Verification items for the finished model (mm, model axes). Face numbers are marked on the shaded views. Give positions to 0.01 mm unless a question says otherwise; leave off trailing zeros. Loops run counter-clockwise (first coordinate to the right, second up) from the corner with the lowest first, then second, coordinate; pieces in that order, holes last. Notation, with made-up numbers: (89, 55) -> (126, 55) arc R23 cw to (126, 64) -> close; hole circle Ø7 at (-19.75, 65). An arc over 180 degrees is marked (long way). Answer in a Markdown table with one row per item. Add a question column.
Q1. Material ranges on probe 1 along X at (y, z) = (16.5, -7.45); probe 2 along Z at (x, y) = (1.5, 26); probe 3 along X at (y, z) = (33, -3.4), recorded low to high.
Q2. Gauge pin test, flat ends, axial feed: P1, Ø3, axis at x = 1, y = 31.5, coming from the -Z side; P2, Ø0.8, axis at x = 0.5, z = -6.5, coming from the -Y side; P3, Ø1.1, axis at x = 6, z = -3.5, coming from the +Y side. Record the tip position at first contact, or that the pin passes through.
Q3. Section check C-C on z = -7.45. Enter the section's corners in (x, y), and give its area (3 significant figures).
Q4. Section check A-A on y = 17. Enter the section's corners in (x, z), and give its area (3 significant figures).
Q5. Section check B-B on x = -9. Enter the section's corners in (y, z).
Q6. Release check for a two-part mould opening along Z. For the marked faces 1 and 2 record: pulls with the +Z half, pulls with the -Z half, needs draft (parallel to the pull), parting line crosses it, or undercut.
```python
from build123d import *

# Parameters (mm, degrees)
SKETCH_W        = 41.5
SKETCH_H        = 36
PAD_DEPTH       = 6
POCKET_DEPTH    = 5
SKETCH002_W     = 19.5
SKETCH002_H     = 8
POCKET001_DEPTH = 6.001
POCKET002_DEPTH = 1
SKETCH005_W     = 1
SKETCH005_H     = 19
PAD001_DEPTH    = 4
PAD002_DEPTH    = 10
SKETCH007_W     = 52.700282
SKETCH007_H     = 20.841337
POCKET003_DEPTH = 41.501
SKETCH008_W     = 1
SKETCH008_H     = 18
PAD003_DEPTH    = 4


with BuildPart() as part:
    # Sketch → Pad (new body)
    with BuildSketch(Plane.XY):
        with Locations((-0.25, 18)):
            Rectangle(SKETCH_W, SKETCH_H)
    extrude(amount=PAD_DEPTH)

    # Sketch001 (on Face6 of Pad) → Pocket (cut)
    with BuildSketch(Plane.XY.offset(6)):
        Polygon((-19, 2), (18.5, 2), (18.5, 26), (-1, 26), (-1, 34), (-19, 34), align=None)
    extrude(amount=-POCKET_DEPTH, mode=Mode.SUBTRACT)

    # Sketch002 (on Face5 of Pocket) → Pocket001 (cut, through all)
    with BuildSketch(Plane.XY.offset(6)):
        with Locations((10.75, 32)):
            Rectangle(SKETCH002_W, SKETCH002_H)
    extrude(amount=-POCKET001_DEPTH, mode=Mode.SUBTRACT)

    # Sketch004 (on Face5 of Pocket001) → Pocket002 (cut)
    with BuildSketch(Plane.XY.offset(6)):
        Polygon((-20, 35), (0, 35), (0, 27), (19.5, 27), (19.5, 1), (-20, 1), align=None)
    extrude(amount=-POCKET002_DEPTH, mode=Mode.SUBTRACT)

    # Sketch005 (on Face22 of Pocket002) → Pad001 (join)
    with BuildSketch(Plane.XY.offset(1)):
        with Locations((-0.5, 16.5)):
            Rectangle(SKETCH005_W, SKETCH005_H)
    extrude(amount=PAD001_DEPTH)

    # Sketch006 (on Face5 of Pad001) → Pad002 (join)
    with BuildSketch(Plane.XY.offset(6)):
        Polygon((-20, 35), (0, 35), (0, 27), (19.5, 27), (19.5, 1), (-20, 1), align=None)
    extrude(amount=-PAD002_DEPTH)

    # Sketch007 (on Face2 of Pad002) → Pocket003 (cut, through all)
    with BuildSketch(Plane(origin=(-21, 0, 0), x_dir=(0, -1, 0), z_dir=(-1, 0, 0))):
        with Locations((-14.885127, 7.420668)):
            Rectangle(SKETCH007_W, SKETCH007_H)
    extrude(amount=-POCKET003_DEPTH, mode=Mode.SUBTRACT)

    # Sketch008 (on Face4 of Pocket003) → Pad003 (join)
    with BuildSketch(Plane(origin=(0, 0, -4), x_dir=(1, 0, 0), z_dir=(0, 0, -1))):
        with Locations((0.5, -16)):
            Rectangle(SKETCH008_W, SKETCH008_H)
    extrude(amount=PAD003_DEPTH)


solid = part.part
```
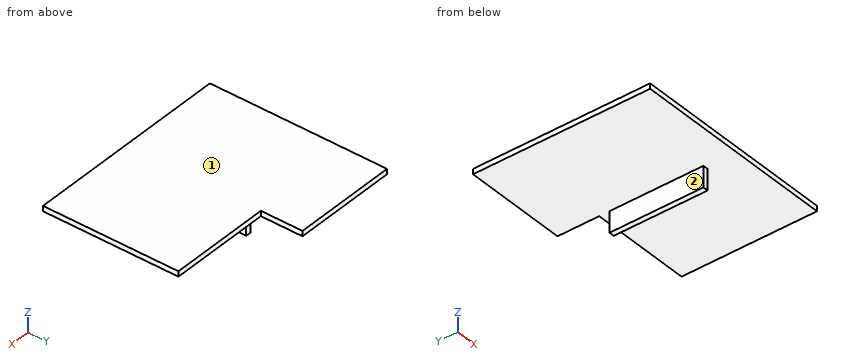
Taken from the geometry:
| question | item | result |
|---|---|---|
| 1 | probe 1 | x = 0 to 1 |
| 1 | probe 2 | z = -4 to -3 |
| 1 | probe 3 | x = -20 to 0 |
| 2 | P1 | stops at z = -4 |
| 2 | P2 | stops at y = 7 |
| 2 | P3 | stops at y = 27 |
| 3 | outline | (0, 7) -> (1, 7) -> (1, 25) -> (0, 25) -> close |
| 3 | area | 18.0 mm² |
| 4 | outline | (-20, -4) -> (0, -4) -> (0, -8) -> (1, -8) -> (1, -4) -> (19.5, -4) -> (19.5, -3) -> (-20, -3) -> close |
| 4 | area | 43.5 mm² |
| 5 | outline | (1, -4) -> (35, -4) -> (35, -3) -> (1, -3) -> close |
| 6 | face 1 | pulls with the +Z half |
| 6 | face 2 | needs draft |
